Geometry check sheet. Reference: the model listing, model coordinates, mm. A direction names the side the tool comes from. Coordinates: 2 decimals unless noted, no trailing zeros. Order: outer loops, then holes, each group sorted by start corner. A loop starts at its lowest first (then second) coordinate and runs counter-clockwise, first axis right, second up. Notation, with made-up numbers: M 21,39.5 L 75,39.5 A27 ccw 75,65.5 Z; hole C 83,41.5 d8. An arc over 180 degrees is marked long. One line per item, written item: value. Start each with the question number.
1) Sectioned sample at A-A, the plane z = 13. Enter the section's corners in (x, y).
2) Sectioned sample at C-C, the plane x = -6. Enter the section's corners in (y, z), then the cut area to 3 significant figures.
3) Sectioned sample at B-B, the plane y = 11. Enter the section's corners in (x, z), then the cut area to 3 significant figures.
4) Go/stop test with flat-tipped pins: P1, Ø3.5, axis at x = 29.37, y = 27.22, coming from the +Z side; P2, Ø1.2, axis at x = 31.5, y = -8.5, coming from the -Z side; P3, Ø2, axis at x = 31.5, z = 4, coming from the +Y side; P4, Ø8.5, axis at x = 14, z = 11, coming from the +Y side. Record where each tip stops, or that it passes through.
5) Thickness scan on L1, parallel to Z at x = -11, y = 2.5; L2, parallel to X at y = -8.4, z = 13; L3, parallel to Y at x = 28.5, z = 20.75. Record the ranges inside material, lowest first. Write a range as from..to.
6) Access from +Z, -Z, +X, -X, +Y, -Y to the whole of each face (thin tool, end or side, straight path). Record for faces 4 (the flat face through (14, 11, 23.5)), 5 (the cylindrical face through (23.376, -8.513, 12.912)).
7) Draft check along X on faces 1 (the cylindrical face through (28.984, 30.194, 1.232)), 2 (the flat face through (-20.625, -9, 13)), 3 (the cylindrical face through (8.78, -6.71, 22.9)). Enter one of: pulls with the +X half, pulls with the -X half, needs draft (parallel to the pull), parting line crosses it, or undercut.
8) Sectioned sample at D-D, the plane x = 4. Enter the section's corners in (y, z).
```python
from build123d import *

# Parameters (mm, degrees)
SKETCH1_R           = 3
BOSS_EXTRUDE1_DEPTH = 26
SHELL1_T            = -2.5
FILLET1_R           = 2
SKETCH2_R           = 4
CUT_EXTRUDE1_DEPTH  = 10.780316569
CUT_EXTRUDE2_DEPTH  = 10.780316569


with BuildPart() as part:
    # Sketch1 → Boss-Extrude1 (new body)
    with BuildSketch(Plane.XY):
        with BuildLine():
            Line((-20.625157389, -9.780316569), (37.374842611, -9.780316569))
            Line((37.374842611, -9.780316569), (37.374842611, 27.219683431))
            ThreePointArc((37.374842611, 27.219683431), (33.242887907, 34.222413298), (25.115286215, 33.991402512))
            Line((25.115286215, 33.991402512), (-20.625157389, 5.219683431))
            Line((-20.625157389, 5.219683431), (-20.625157389, -9.780316569))
        make_face()
        with Locations((29.374842611, 27.219683431)):
            Circle(SKETCH1_R, mode=Mode.SUBTRACT)
    extrude(amount=BOSS_EXTRUDE1_DEPTH)

    # Shell1
    shell1_openings = [part.faces().sort_by_distance(p)[0] for p in [
        (2.245064413, 19.605542972, 13),
        (32.24397616, 32.413978135, 13),
        (37.374842611, 8.719683431, 13),
        (-20.625157389, -2.280316569, 13),
        (32.374842611, 27.219683431, 26),
    ]]
    offset(amount=SHELL1_T, openings=shell1_openings, kind=Kind.INTERSECTION)

    # Fillet1
    fillet1_edges = [part.edges().sort_by_distance(p)[0] for p in [
        (-20.625157389, 5.219683431, 1.25),
        (8.374842611, -7.280316569, 23.5),
        (8.374842611, -7.280316569, 2.5),
        (8.374842611, -9.780316569, 0),
        (8.374842611, -9.780316569, 26),
        (-20.625157389, 5.219683431, 24.75),
    ]]
    fillet(fillet1_edges, radius=FILLET1_R)

    # Sketch2 → Cut-Extrude1 (cut, through all)
    with BuildSketch(Plane(origin=(0, 0, 0), x_dir=(1, 0, 0), z_dir=(0, 1, 0))):
        with Locations((-8.625157389, -13)):
            Circle(SKETCH2_R)
    extrude(amount=-CUT_EXTRUDE1_DEPTH, mode=Mode.SUBTRACT)

    # Sketch3 → Cut-Extrude2 (cut, through all)
    with BuildSketch(Plane(origin=(0, 0, 0), x_dir=(1, 0, 0), z_dir=(0, 1, 0))):
        with BuildLine():
            Line((37.374842611, -9), (27.374842611, -9))
            ThreePointArc((27.374842611, -9), (23.374842611, -13), (27.374842611, -17))
            Line((27.374842611, -17), (37.374842611, -17))
            Line((37.374842611, -17), (37.374842611, -9))
        make_face()
    extrude(amount=-CUT_EXTRUDE2_DEPTH, mode=Mode.SUBTRACT)


solid = part.part
```
Final values:
1. outline: M -20.63,-9.78 L -12.63,-9.78 L -12.63,-7.28 L -20.63,-7.28 Z; M -4.63,-9.78 L 23.37,-9.78 L 23.37,-7.28 L -4.63,-7.28 Z
2. outline: M -9.78,2 A2 ccw -7.78,0 L 14.42,0 L 14.42,2.5 L -5.28,2.5 A2 cw -7.28,4.5 L -7.28,9.98 L -9.78,9.98 Z; M -9.78,16.02 L -7.28,16.02 L -7.28,21.5 A2 cw -5.28,23.5 L 14.42,23.5 L 14.42,26 L -7.78,26 A2 ccw -9.78,24 Z
2. area: 158 mm^2
3. outline: M -11.44,0 L 37.37,0 L 37.37,2.5 L -11.44,2.5 Z; M -11.44,23.5 L 37.37,23.5 L 37.37,26 L -11.44,26 Z
3. area: 244 mm^2
4. P1: passes through
4. P2: stops at z = 0
4. P3: stops at y = -6.6
4. P4: stops at y = -7.28
5. L1: z = 0..2.5, 23.5..26
5. L2: x = -20.63..-12.63, -4.63..23.37
5. L3: y = -9.78..-7.28
6. face 4: +X, -X, +Y
6. face 5: +X, +Y, -Y
7. face 1: undercut
7. face 2: pulls with the -X half
7. face 3: needs draft
8. outline: M -9.78,2 A2 ccw -7.78,0 L 20.71,0 L 20.71,2.5 L -5.28,2.5 A2 cw -7.28,4.5 L -7.28,21.5 A2 cw -5.28,23.5 L 20.71,23.5 L 20.71,26 L -7.78,26 A2 ccw -9.78,24 Z
